Geometry check sheet. Reference: drawing and pictorial views, mm from the part's lowest x, y, z. A direction names the side the tool comes from. Give positions to 0.01 mm unless a question says otherwise; leave off trailing zeros. Order: outer loops, then holes, each group sorted by start corner. A loop starts at its lowest first (then second) coordinate and runs counter-clockwise, first axis right, second up.
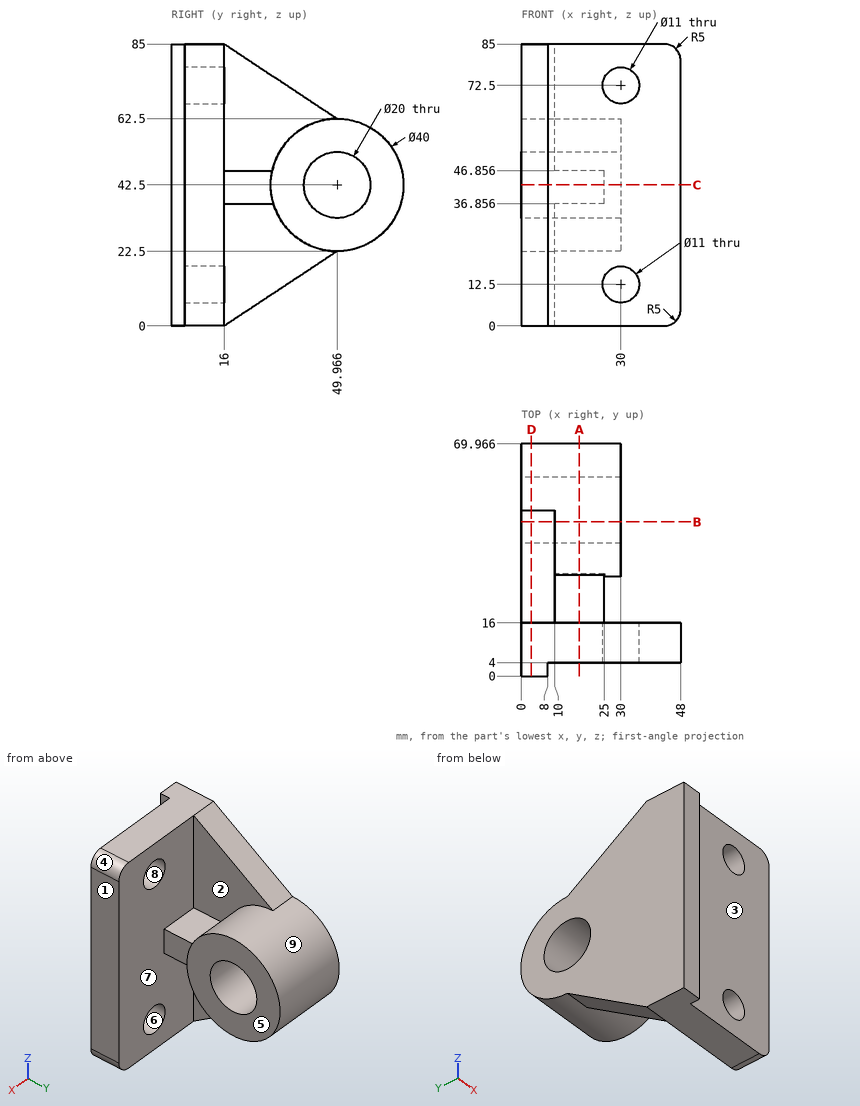
1) Material ranges on L1, parallel to X at y = 10, z = 72.5; L2, parallel to Y at x = 28, z = 49.5; L3, parallel to Z at x = 30.5, y = 7.5, recorded low to high.
Recorded:
L1: x = 0 to 24.5, 35.5 to 48
L2: y = 4 to 16, 31.23 to 42.82, 57.11 to 68.7
L3: z = 0 to 7.02, 17.98 to 67.02, 77.98 to 85
2) Section check D-D, the plane x = 3. Record the cut outline in (y, z).
Recorded:
outline: (0, 0) - (16, 0) - (49.97, 22.5) arc R20 ccw to (49.97, 62.5) - (16, 85) - (0, 85) - close; hole circle Ø20 at (49.97, 42.5)
3) Section check C-C, the plane z = 42.5. Record the cut outline in (x, y), then the cut area to 3 significant figures.
Recorded:
outline: (0, 0) - (8, 0) - (8, 4) - (48, 4) - (48, 16) - (25, 16) - (25, 29.97) - (30, 29.97) - (30, 39.97) - (0, 39.97) - close; (0, 59.97) - (30, 59.97) - (30, 69.97) - (0, 69.97) - close
area: 1,560 mm2
4) Section check A-A, the plane x = 17.5. Record the cut outline in (y, z), then the cut area to 3 significant figures.
Recorded:
outline: (4, 0) - (16, 0) - (16, 36.86) - (30.78, 36.86) arc R20 ccw (long way) to (30.45, 46.86) - (16, 46.86) - (16, 85) - (4, 85) - close; hole circle Ø20 at (49.97, 42.5)
area: 2,100 mm2
5) Depth check by flat-ended pin: pin 1 Ø6 at (x, z) = (36.5, 55.5) entering from -Y; pin 2 Ø11 at (y, z) = (22, 42.5) entering from +X; pin 3 Ø14.5 at (x, z) = (30, 72.5) entering from +Y. Enter the tip coordinate at first touch or a pass-through.
Recorded:
pin 1: stops at y = 4
pin 2: stops at x = 25
pin 3: stops at y = 16
6) Section check B-B, the plane y = 46.5. Record the cut outline in (x, z).
Recorded:
outline: (0, 20.2) - (10, 20.2) - (10, 22.8) - (30, 22.8) - (30, 33.12) - (0, 33.12) - close; (0, 51.88) - (30, 51.88) - (30, 62.2) - (10, 62.2) - (10, 64.8) - (0, 64.8) - close
7) Draft check along Z on the marked faces 6, 7, 8 and 9. Enter one of: +Z half, -Z half, draft (parallel to the pull), parting line (faces both ways), or undercut.
Recorded:
face 6: undercut
face 7: draft
face 8: undercut
face 9: parting line
8) Set-up check for the marked faces 1, 2, 3, 4 and 5: record each of +Z, -Z, +X, -X, +Y, -Y from which the full face is reachable in a straight line by a thin tool's end or side.
Recorded:
face 1: +Z, -Z, +X, +Y, -Y
face 2: +Z, +X
face 3: +Z, -Z, +X, -Y
face 4: +Z, +X, +Y, -Y
face 5: +Z, -Z, +X, +Y
